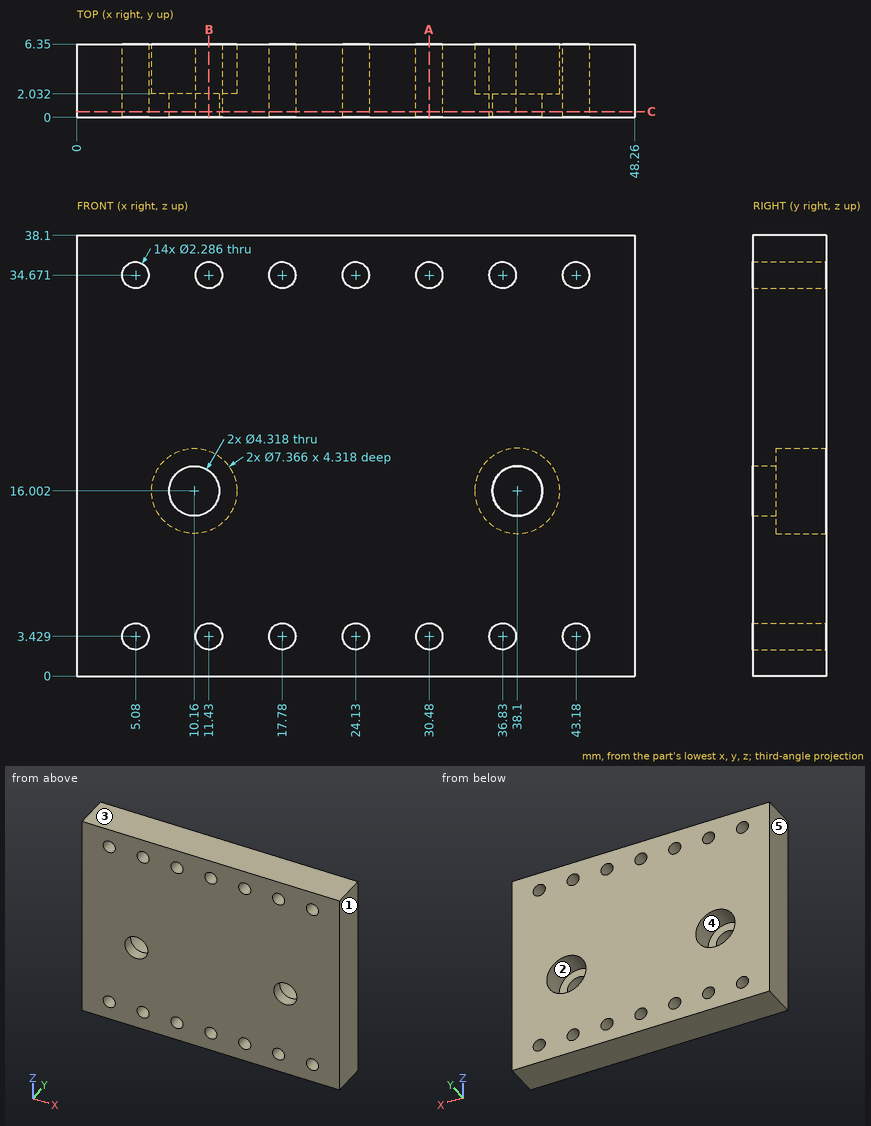
Drawing for the job (mm, zero at the part's lowest x, y, z). A direction names the side the tool comes from. Coordinates: 2 decimals unless noted, no trailing zeros. Loops run counter-clockwise (first coordinate to the right, second up) from the corner with the lowest first, then second, coordinate; pieces in that order, holes last. Notation, with made-up numbers: (54.5, 62.5) - (96.5, 62.5) arc R33 cw to (96.5, 91.5) - close; hole circle Ø10 at (49, 22). An arc over 180 degrees is marked (long way). Use CSV: the item, a comma, the result in double quotes. Start each with the question number.
Q1. Cut at B-B, the plane x = 11.43. List the corners of the cut face in (y, z).
Q2. 3-axis set-ups, long thin cutter, end or side, ignore diameter. For the marked faces 1 and 2: which of +Z, -Z, +X, -X, +Y, -Y reach the whole face in a straight line?
Q3. Two-plate mould, pull along X, no slides. Class the marked faces 3, 4 and 5: +X half, -X half, draft (parallel to the pull), parting line (faces both ways), or undercut.
Q4. Cut at A-A, the plane x = 30.48. List the corners of the cut face in (y, z), then the cut area to 3 significant figures.
Q5. Probe probe 1 along Z at (x, y) = (17.78, 3.75); probe 2 along Z at (x, y) = (10.16, 5.3) (3 decimals); probe 3 along Z at (x, y) = (6, 4.5). List the from-to ranges inside material, lowest first. Write a range as from..to.
Q6. Cut at C-C, the plane y = 0.5. State how many separate pieces and enclosed holes the cut face has, then the cut area to 3 significant figures.
Q7. Drop a flat-ended pin along its axis: P1, Ø3.5, axis at x = 11, z = 17, coming from the +Y side. Give the stop position or say it passes through.
Here are the results:
1,outline,"(0, 0) - (6.35, 0) - (6.35, 2.29) - (0, 2.29) - close; (0, 4.57) - (6.35, 4.57) - (6.35, 12.54) - (2.03, 12.54) - (2.03, 14.26) - (0, 14.26) - close; (0, 17.75) - (2.03, 17.75) - (2.03, 19.46) - (6.35, 19.46) - (6.35, 33.53) - (0, 33.53) - close; (0, 35.81) - (6.35, 35.81) - (6.35, 38.1) - (0, 38.1) - close"
2,face 1,"+Z, -Z, +X, +Y, -Y"
2,face 2,"+Y"
3,face 3,"draft"
3,face 4,"undercut"
3,face 5,"-X half"
4,outline,"(0, 0) - (6.35, 0) - (6.35, 2.29) - (0, 2.29) - close; (0, 4.57) - (6.35, 4.57) - (6.35, 33.53) - (0, 33.53) - close; (0, 35.81) - (6.35, 35.81) - (6.35, 38.1) - (0, 38.1) - close"
4,area,"213 mm2"
5,probe 1,"0..2.29, 4.57..33.53, 35.81..38.1"
5,probe 2,"0..12.319, 19.685..38.1"
5,probe 3,"0..2.75, 4.11..33.99, 35.35..38.1"
6,separate pieces,"1"
6,enclosed holes,"16"
6,area,"1,750 mm2"
7,P1,"y = 2.03"
